```python
from build123d import *

# Parameters (mm, degrees)
F1_DEPTH  = 63.5
F2_DEPTH  = 25.4
F3_DEPTH  = 7.9375
F2_FACE_W = 50.8
F2_FACE_H = 19.05
F4_DEPTH  = 25.4
F7_R      = 5.08
F8_R      = 6.35


with BuildPart() as f1:
    # F0 (on Front) → F1 (new body, symmetric)
    with BuildSketch(Plane.XZ):
        Polygon((22.225, 9.525), (-41.275, 9.525), (-41.275, -9.525), (41.275, -9.525), (41.275, 9.525), align=None)
    extrude(amount=F1_DEPTH, both=True)

    # F0 (on Front) → F2 (join, symmetric)
    with BuildSketch(Plane.XZ):
        with BuildLine():
            Line((22.225, 27.0002), (22.225, 9.525))
            Line((22.225, 9.525), (41.275, 9.525))
            Line((41.275, 9.525), (41.275, 27.0002))
            ThreePointArc((41.275, 27.0002), (45.92468, 38.22552), (57.15, 42.8752))
            Line((57.15, 42.8752), (60.325, 42.8752))
            Line((60.325, 42.8752), (60.325, 61.9252))
            Line((60.325, 61.9252), (57.15, 61.9252))
            add(Edge.make_bspline(
                [(56.663359, 61.921809), (56.825525, 61.923217), (56.987739, 61.924347), (57.15, 61.9252)],
                knots=[111.064005, 111.064005, 111.064005, 111.064005, 111.504536, 111.504536, 111.504536, 111.504536], degree=3))
            ThreePointArc((56.663359, 61.921809), (32.282837, 51.523247), (22.225, 27.0002))
        make_face()
    extrude(amount=F2_DEPTH, both=True)

    # F0 (on Front) → F3 (join, symmetric)
    with BuildSketch(Plane.XZ):
        with BuildLine():
            add(Edge.make_bspline(
                [(-41.275, 9.525), (-22.040929, 43.59531), (15.779117, 61.566989), (56.663359, 61.921809)],
                knots=[0, 0, 0, 0, 111.064005, 111.064005, 111.064005, 111.064005], degree=3))
            Line((-41.275, 9.525), (22.225, 9.525))
            Line((22.225, 9.525), (22.225, 27.0002))
            ThreePointArc((22.225, 27.0002), (32.282837, 51.523247), (56.663359, 61.921809))
        make_face()
    extrude(amount=F3_DEPTH, both=True)

    # F2_face (on face) → F4 (join)
    with BuildSketch(Plane(origin=(60.325, 0, 52.4002), x_dir=(0, 1, 0), z_dir=(1, 0, 0))):
        Rectangle(F2_FACE_W, F2_FACE_H)
    extrude(amount=F4_DEPTH)

    # F0 (on Front) → F6 (revolve)
    with BuildSketch(Plane.XZ):
        Polygon((85.725, 66.675), (85.725, 61.9252), (85.725, 42.8752), (85.725, 38.1), (111.125, 38.1), (111.125, 66.675), align=None)
    revolve(axis=Axis((85.725, 0, 52.3875), (0, 0, -1)))

    # F7
    f7_edges = [f1.edges().sort_by_distance(p)[0] for p in [
        (41.275, -63.5, 0),
        (41.275, 63.5, 0),
        (-41.275, 63.5, 0),
    ]]
    fillet(f7_edges, radius=F7_R)

    # F8
    f8_edges = [f1.edges().sort_by_distance(p)[0] for p in [
        (-41.275, -63.5, 0),
    ]]
    fillet(f8_edges, radius=F8_R)


solid = f1.part
```
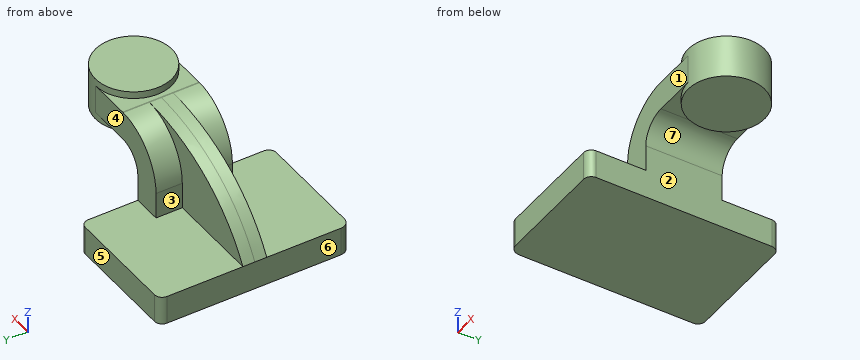
Source: CAD feature listing. Evaluate the final solid. Frame: model axes, mm. Face numbers are marked on the shaded views. A direction names the side the tool comes from. Give positions to 0.01 mm unless a question says otherwise; leave off trailing zeros. Write each loop counter-clockwise with the first axis right and the second up, starting at its lowest first coordinate (ties: lowest second). Pieces come first, ordered by that corner, then holes.
1. Material intervals for line 1 along Z through (x, y) = (17.5, 17) (3 decimals); line 2 along Y through (x, z) = (10, 24); line 3 along Y through (x, z) = (41, 44), sorted ascending.
2. Pull-direction query (X, two-part tool) for the marked faces 5, 6 and 7; classes: +X half, -X half, draft (parallel to the pull), parting line (faces both ways), or undercut.
3. Section query A-A (z = 1). Return the cut outline in (x, y) (3 decimals).
4. First-contact query: pin 1 (14 mm diameter, centred on y = -13.5, z = 21.5, fed in from -X); pin 2 (5 mm diameter, centred on x = 73, y = -12, fed in from -Z); pin 3 (2 mm diameter, centred on y = 5.5, z = 16.5, fed in from -X). Flat tips, straight axial feed; report the tip coordinate or a pass-through.
5. Access query for the marked faces 1, 2, 3 and 4. Directions: +Z, -Z, +X, -X, +Y, -Y. A direction counts if a zero-diameter tool reaches every point of the face in a straight line with its end or side. Return the directions, or none.
6. Section query C-C (y = 51). Return the cut outline in (x, z) (3 decimals).
7. Section query B-B (x = 75). Return the cut outline in (y, z) (3 decimals).
Output values:
1. line 1: z = -9.525 to 9.525
1. line 2: y = -7.94 to 7.94
1. line 3: y = -25.4 to 25.4
2. face 5: draft
2. face 6: -X half
2. face 7: undercut
3. outline: (-41.275, -57.15) arc R6.35 ccw to (-34.925, -63.5) - (36.195, -63.5) arc R5.08 ccw to (41.275, -58.42) - (41.275, 58.42) arc R5.08 ccw to (36.195, 63.5) - (-36.195, 63.5) arc R5.08 ccw to (-41.275, 58.42) - close
4. pin 1: stops at x = -36.41
4. pin 2: stops at z = 38.1
4. pin 3: stops at x = -37.6
5. face 1: +Z, +X, -X, -Y
5. face 2: -Z, +X, +Y, -Y
5. face 3: +Z, -X, +Y
5. face 4: +Z, +X, -X, +Y
6. outline: (-41.275, -9.525) - (41.275, -9.525) - (41.275, 9.525) - (-41.275, 9.525) - close
7. outline: (-25.4, 42.875) - (-23.025, 42.875) - (-23.025, 38.1) - (23.025, 38.1) - (23.025, 42.875) - (25.4, 42.875) - (25.4, 61.925) - (23.025, 61.925) - (23.025, 66.675) - (-23.025, 66.675) - (-23.025, 61.925) - (-25.4, 61.925) - close
